from build123d import *

# Parameters (mm, degrees)
SKETCH1_W             = 80
SKETCH1_H             = 21.75
MAIN_DEPTH            = 8
M5_CLEARANCE_HOLE1_D  = 5.5
F_2_CLEARANCE_HOLE1_D = 2.2606
SPACER_DEPTH          = 8
CUT_EXTRUDE3_DEPTH    = 10
CHAMFER1_SIZE         = 5
FILLET1_R             = 2.5


with BuildPart() as part:
    # Sketch1 → Main (new body)
    with BuildSketch(Plane(origin=(0, 0, 0), x_dir=(0, 0, -1), z_dir=(1, 0, 0))):
        Rectangle(SKETCH1_W, SKETCH1_H)
    extrude(amount=MAIN_DEPTH)

    # M5 Clearance Hole1 (through all)
    with Locations(Plane.ZY):
        with Locations((-20, 1.625), (33.5, 1.625)):
            Hole(M5_CLEARANCE_HOLE1_D / 2)

    # #2 Clearance Hole1 (through all)
    with Locations(Plane.ZY):
        with Locations((0, -8.375), (0, 4.325)):
            Hole(F_2_CLEARANCE_HOLE1_D / 2)

    # Sketch13 → Spacer (add)
    with BuildSketch(Plane.ZY):
        Polygon((40, 10.875), (47.5, 10.875), (47.5, -15.875), (-47.5, -15.875), (-47.5, 10.875), (-40, 10.875), (-40, -10.875), (40, -10.875), align=None)
    extrude(amount=-SPACER_DEPTH)

    # Sketch14 → Cut-Extrude3 (cut)
    with BuildSketch(Plane.ZY):
        with BuildLine():
            Line((38.5, -1.125), (28.5, -1.125))
            ThreePointArc((28.5, -1.125), (25.75, 1.625), (28.5, 4.375))
            Line((28.5, 4.375), (38.5, 4.375))
            ThreePointArc((38.5, 4.375), (41.25, 1.625), (38.5, -1.125))
        make_face()
        with BuildLine():
            Line((-15, -1.125), (-25, -1.125))
            ThreePointArc((-25, -1.125), (-27.75, 1.625), (-25, 4.375))
            Line((-25, 4.375), (-15, 4.375))
            ThreePointArc((-15, 4.375), (-12.25, 1.625), (-15, -1.125))
        make_face()
        with BuildLine():
            Line((1.1303, -5.875), (1.1303, -10.875))
            ThreePointArc((1.1303, -10.875), (0, -12.0053), (-1.1303, -10.875))
            Line((-1.1303, -10.875), (-1.1303, -5.875))
            ThreePointArc((-1.1303, -5.875), (0, -4.7447), (1.1303, -5.875))
        make_face()
        with BuildLine():
            Line((1.1303, 6.825), (1.1303, 1.825))
            ThreePointArc((1.1303, 1.825), (0, 0.6947), (-1.1303, 1.825))
            Line((-1.1303, 1.825), (-1.1303, 6.825))
            ThreePointArc((-1.1303, 6.825), (0, 7.9553), (1.1303, 6.825))
        make_face()
    extrude(amount=-CUT_EXTRUDE3_DEPTH, mode=Mode.SUBTRACT)

    # Chamfer1
    chamfer1_edges = [part.edges().sort_by_distance(p)[0] for p in [
        (4, 10.875, -47.5),
        (4, 10.875, 47.5),
        (4, -15.875, 47.5),
        (4, -15.875, -47.5),
    ]]
    chamfer(chamfer1_edges, length=CHAMFER1_SIZE)

    # Fillet1
    fillet1_edges = [part.edges().sort_by_distance(p)[0] for p in [
        (4, 10.875, 42.5),
        (4, 10.875, -42.5),
        (4, -10.875, -47.5),
        (4, 5.875, -47.5),
        (4, -15.875, 42.5),
        (4, -15.875, -42.5),
        (4, -10.875, 47.5),
        (4, 5.875, 47.5),
    ]]
    fillet(fillet1_edges, radius=FILLET1_R)


solid = part.part
Can you work these out from the model? Positions are in its coordinate system, mm. A direction names the side the tool comes from. Coordinates: 2 decimals unless noted, no trailing zeros. Loops run counter-clockwise (first coordinate to the right, second up) from the corner with the lowest first, then second, coordinate; pieces in that order, holes last. Notation, with made-up numbers: (-2, 70) - (4, 70) arc R18 ccw to (4, 103) - close; hole circle Ø3 at (41.25, 18.5). An arc over 180 degrees is marked (long way). Answer as a JSON object with one key per item and string values. Group by question number.
Item 1: On a 3-axis mill with a long thin cutter (end or side, diameter ignored), from which of +Z, -Z, +X, -X, +Y, -Y can I reach the whole of each face in a straight line? I mean faces 5 (the face through (3.94, 1.56, 25.75)), 6 (the face through (4.06, -15.68, 42.43)). Say none if no direction works.
Item 2: If we mould it in two halves opening along Z, with no side actions, what happens to faces 1 (the face through (3.944, -12.005, 0.025)), 2 (the face through (4.06, 10.69, -42.41)), 3 (the face through (3.944, -13.35, 45.025)), 4 (the face through (4, 10.875, -1))? For each: released by +Z, released by -Z, zero draft, split by the parting line, or undercut.
Item 3: If I drill on L1, parallel to Z at x = 0.5, y = 1.75; L2, parallel to Y at x = 4.25, z = -20.5 (3 decimals); L3, parallel to Z at x = 5.75, y = -9, over which ranges is the centre line in solid material (lowest first)? Write a range as from..to.
Item 4: If we section it at B-B (x = 5.25): State how many separate pieces and enclosed holes the cut face has, plus the area to 3 significant figures.
Item 5: If we section it at D-D (y = 3.5): List the corners of the cut face in (x, z) for me.
Item 6: If we section it at C-C (z = 0): List the corners of the cut face in (x, y) for me (3 decimals).
Item 7: If we section it at A-A (z = -20): List the corners of the cut face in (x, y) for me (3 decimals), plus the area to 3 significant figures.
Returned:
{
 "1": {"face 5": "+X, -X", "face 6": "+Z, +X, -X, -Y"},
 "2": {"face 1": "undercut", "face 2": "released by -Z", "face 3": "released by +Z", "face 4": "zero draft"},
 "3": {"L1": "z = -47.5..-27.75, -12.25..-1.13, 1.13..25.75, 41.25..47.5", "L2": "y = -15.875..-1.125, 4.375..10.875", "L3": "z = -47.5..-1.13, 1.13..47.5"},
 "4": {"separate pieces": "1", "enclosed holes": "4", "area": "2,300 mm²"},
 "5": {"outline": "(0, -47.5) - (8, -47.5) - (8, -27.01) - (0, -27.01) - close; (0, -12.99) - (8, -12.99) - (8, -1.13) - (0, -1.13) - close; (0, 1.13) - (8, 1.13) - (8, 26.49) - (0, 26.49) - close; (0, 40.51) - (8, 40.51) - (8, 47.5) - (0, 47.5) - close"},
 "6": {"outline": "(0, -15.875) - (8, -15.875) - (8, -12.005) - (0, -12.005) - close; (0, -4.745) - (8, -4.745) - (8, 0.695) - (0, 0.695) - close; (0, 7.955) - (8, 7.955) - (8, 10.875) - (0, 10.875) - close"},
 "7": {"outline": "(0, -15.875) - (8, -15.875) - (8, -1.125) - (0, -1.125) - close; (0, 4.375) - (8, 4.375) - (8, 10.875) - (0, 10.875) - close", "area": "170 mm²"}
}
